Geometry check sheet. Reference: drawing and pictorial views, mm from the part's lowest x, y, z. A direction names the side the tool comes from. Give positions to 0.01 mm unless a question says otherwise; leave off trailing zeros. Order: outer loops, then holes, each group sorted by start corner. A loop starts at its lowest first (then second) coordinate and runs counter-clockwise, first axis right, second up. Notation, with made-up numbers: (63.25, 11.25) -> (77.25, 11.25) arc R14 cw to (77.25, 36.25) -> close; hole circle Ø3 at (48, -6.5). An arc over 180 degrees is marked (long way). Write each question's results on one line, items separated by ' | '.
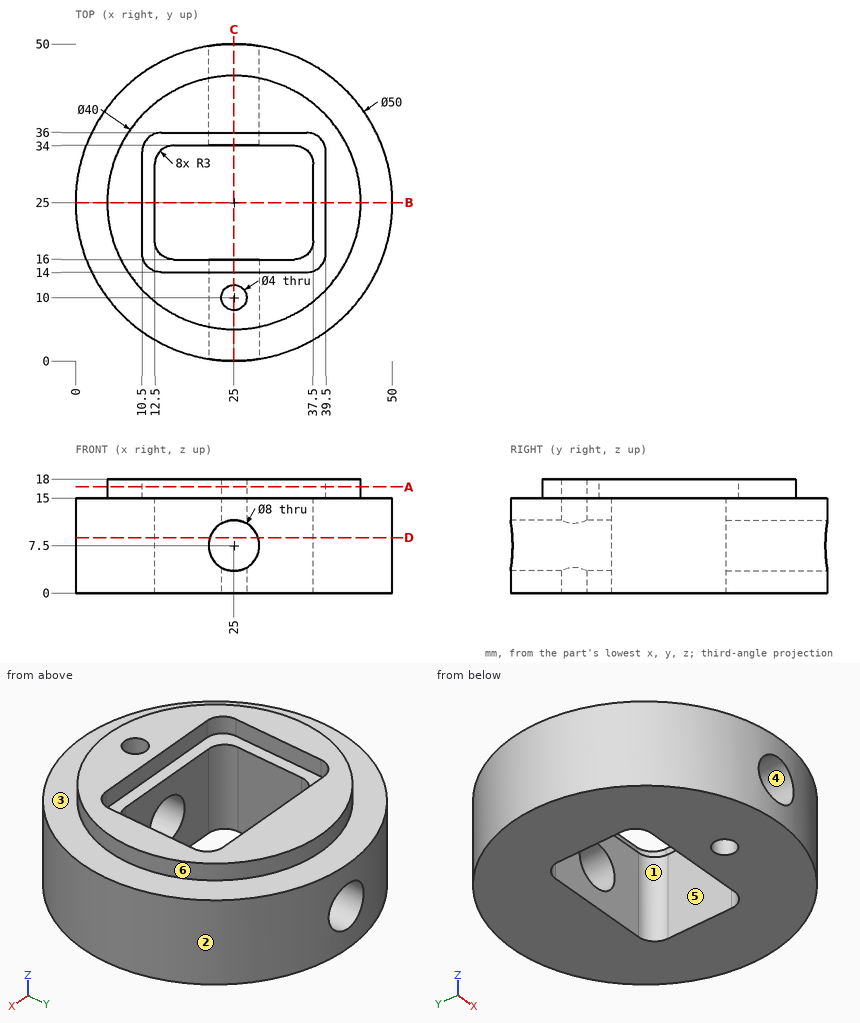
1. Mould release check, pull along Y, two halves, no side actions. Record for the marked faces 1, 2 and 3: +Y half, -Y half, draft (parallel to the pull), parting line (faces both ways), or undercut.
Verdict:
face 1: undercut | face 2: parting line | face 3: draft
2. Section check C-C on x = 25. Give the number of separate pieces and of enclosed holes in the cut face, then the cut area to 3 significant figures.
Verdict:
separate pieces: 6 | enclosed holes: 0 | area: 238 mm^2
3. Section check B-B on y = 25. Record the cut outline in (x, z).
Verdict:
outline: (0, 0) -> (12.5, 0) -> (12.5, 15) -> (10.5, 15) -> (10.5, 18) -> (5, 18) -> (5, 15) -> (0, 15) -> close; (37.5, 0) -> (50, 0) -> (50, 15) -> (45, 15) -> (45, 18) -> (39.5, 18) -> (39.5, 15) -> (37.5, 15) -> close
4. Section check D-D on z = 8.75. Record the cut outline in (x, y), then the cut area to 3 significant figures.
Verdict:
outline: (12.5, 19) -> (12.5, 31) arc R3 cw to (15.5, 34) -> (21.2, 34) -> (21.2, 49.71) arc R25 ccw to (21.2, 0.29) -> (21.2, 16) -> (15.5, 16) arc R3 cw to start; (28.8, 0.29) arc R25 ccw to (28.8, 49.71) -> (28.8, 34) -> (34.5, 34) arc R3 cw to (37.5, 31) -> (37.5, 19) arc R3 cw to (34.5, 16) -> (28.8, 16) -> close | area: 1,280 mm^2
5. Gauge pin test, flat ends, axial feed: pin 1 Ø0.9 at (x, z) = (29.5, 16.5) entering from -Y; pin 2 Ø10 at (y, z) = (9.5, 10.5) entering from -X; pin 3 Ø2.5 at (x, z) = (21.5, 16) entering from +Y; pin 4 Ø2.5 at (x, y) = (25, 10) entering from -Z. Record the tip position at first contact, or that the pin passes through.
Verdict:
pin 1: stops at y = 5.41 | pin 2: stops at x = 2.31 | pin 3: stops at y = 49.85 | pin 4: passes through
6. Access from +Z, -Z, +X, -X, +Y, -Y to the whole of each face (thin tool, end or side, straight path). Record for the marked faces 4, 5 and 6.
Verdict:
face 4: +Y, -Y | face 5: +Z, -Z | face 6: +Z
7. Material ranges on probe 1 along Y at (x, z) = (25, 1.9); probe 2 along X at (y, z) = (25.5, 15.75); probe 3 along Z at (x, y) = (25, 39), recorded low to high. Write a range as from..to.
Verdict:
probe 1: y = 0..8, 12..16, 34..50 | probe 2: x = 5.01..10.5, 39.5..44.99 | probe 3: z = 0..3.5, 11.5..18
8. Section check A-A on z = 16.75. Record the cut outline in (x, y), then the cut area to 3 significant figures.
Verdict:
outline: circle Ø40 at (25, 25); hole (10.5, 17) arc R3 ccw to (13.5, 14) -> (36.5, 14) arc R3 ccw to (39.5, 17) -> (39.5, 33) arc R3 ccw to (36.5, 36) -> (13.5, 36) arc R3 ccw to (10.5, 33) -> close; hole circle Ø4 at (25, 10) | area: 614 mm^2
